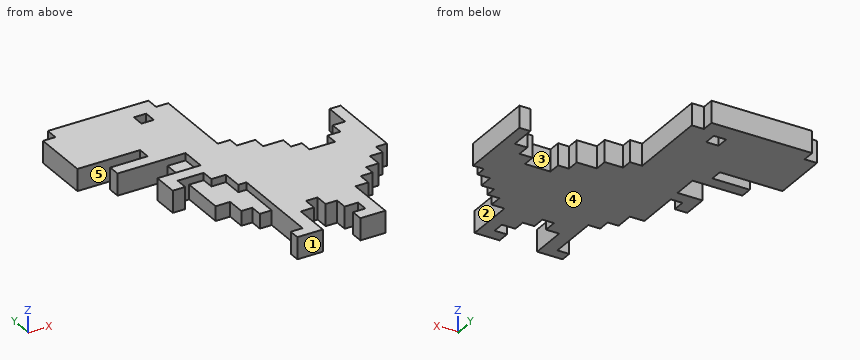
Autodesk Fusion 360 part; units mm, degrees
sketch "Dino" plane through (0, 0, 0) normal (0, 0, 1) x (1, 0, 0)
  line L0 (16.5, 0) -> (20, 0)
  line L1 (20, 0) -> (20, 5)
  line L2 (20, 5) -> (21.8166, 5)
  line L3 (21.8166, 5) -> (21.8166, 6.8132)
  line L4 (21.8166, 6.8132) -> (23.4038, 6.8132)
  line L5 (23.4038, 6.8132) -> (23.4038, 5)
  line L6 (23.4038, 5) -> (25, 5)
  line L7 (25, 5) -> (25, 3.315)
  line L8 (25, 3.315) -> (26.8534, 3.315)
  line L9 (26.8534, 3.315) -> (26.8534, 1.6631)
  line L10 (26.8534, 1.6631) -> (25.1529, 1.6631)
  line L11 (25.1529, 1.6631) -> (25.1529, 0)
  line L12 (25.1529, 0) -> (28.5781, 0)
  line L13 (28.5781, 0) -> (28.5781, 6.758)
  line L14 (28.5781, 6.758) -> (30.3565, 6.758)
  line L15 (30.3565, 6.758) -> (30.3565, 8.5127)
  line L16 (30.3565, 8.5127) -> (32, 8.5127)
  line L17 (32, 8.5127) -> (32, 10)
  line L18 (32, 10) -> (33.7351, 10)
  line L19 (33.7351, 10) -> (33.7351, 12)
  line L20 (33.7351, 12) -> (35.5, 12)
  line L21 (35.5, 12) -> (35.5, 13.5)
  line L22 (35.5, 13.5) -> (37, 13.5)
  line L23 (37, 13.5) -> (37, 24)
  line L24 (37, 24) -> (35.5, 24)
  line L25 (35.5, 24) -> (35.5, 20.5)
  line L26 (35.5, 20.5) -> (33.7869, 20.5)
  line L27 (33.7869, 20.5) -> (33.7869, 18.75)
  line L28 (33.7869, 18.75) -> (32, 18.75)
  line L29 (32, 18.75) -> (32, 17.0258)
  line L30 (32, 17.0258) -> (28.5, 17.0258)
  line L31 (28.5, 17.0258) -> (28.5, 18.75)
  line L32 (28.5, 18.75) -> (27, 18.75)
  line L33 (27, 18.75) -> (27, 20.5)
  line L34 (27, 20.5) -> (24.2282, 20.5)
  line L35 (24.2282, 20.5) -> (24.2282, 22.2618)
  line L36 (24.2282, 22.2618) -> (21.6914, 22.2618)
  line L37 (21.6914, 22.2618) -> (21.6914, 23.7839)
  line L38 (21.6914, 23.7839) -> (20, 23.7839)
  line L39 (20, 23.7839) -> (20, 35)
  line L40 (20, 35) -> (18.3225, 35)
  line L41 (18.3225, 35) -> (18.3225, 36.7116)
  line L42 (18.3225, 36.7116) -> (4.5, 36.7116)
  line L43 (4.5, 36.7116) -> (4.5, 35)
  line L44 (4.5, 35) -> (2.7971, 35)
  line L45 (2.7971, 35) -> (2.7971, 27.2137)
  line L46 (2.7971, 27.2137) -> (11.4112, 27.2137)
  line L47 (11.4112, 27.2137) -> (11.4112, 25.5)
  line L48 (11.4112, 25.5) -> (6.2675, 25.5)
  line L49 (6.2675, 25.5) -> (6.2675, 23.8448)
  line L50 (6.2675, 23.8448) -> (13.127, 23.8448)
  line L51 (13.127, 23.8448) -> (13.127, 20.4572)
  line L52 (13.127, 20.4572) -> (9.6973, 20.4572)
  line L53 (9.6973, 20.4572) -> (9.6973, 17)
  line L54 (9.6973, 17) -> (11.4121, 17)
  line L55 (11.4121, 17) -> (11.4121, 18.7286)
  line L56 (11.4121, 18.7286) -> (13, 18.7286)
  line L57 (13, 18.7286) -> (13, 12.7374)
  line L58 (13, 12.7374) -> (15, 12.7374)
  line L59 (15, 12.7374) -> (15, 10.206)
  line L60 (15, 10.206) -> (16.5, 10.206)
  line L61 (16.5, 10.206) -> (16.5, 8.5)
  line L62 (16.5, 8.5) -> (18.1296, 8.5)
  line L63 (18.1296, 8.5) -> (18.1296, 1.5)
  line L64 (18.1296, 1.5) -> (16.5, 1.5)
  line L65 (16.5, 1.5) -> (16.5, 0)
  line L66 (13.127, 23.8448) -> (15.6157, 23.8448)
  line L67 (15.6157, 23.8448) -> (15.6157, 20.4572)
  line L68 (15.6157, 20.4572) -> (13.127, 20.4572)
  line L69 (13, 18.7286) -> (15, 18.7286)
  line L70 (15, 18.7286) -> (15, 17)
  line L71 (15, 17) -> (17, 17)
  line L72 (17, 17) -> (17, 14.1994)
  line L73 (17, 14.1994) -> (18.1296, 14.1994)
  line L74 (18.1296, 14.1994) -> (18.1296, 8.5)
  line L75 (14.802, 34.2204) -> (14.802, 32.5)
  line L76 (14.802, 32.5) -> (16.5, 32.5)
  line L77 (16.5, 32.5) -> (16.5, 34.2204)
  line L78 (16.5, 34.2204) -> (14.802, 34.2204)
extrude "Extrude1" add sketch "Dino" along normal blind 3 contours L0 L1 L2 L3 L4 L5 L6 L7 L8 L9 L10 L11 L12 L13 L14 L15 L16 L17 L18 L19 L20 L21 L22 L23 L24 L25 L26 L27 L28 L29 L30 L31 L32 L33 L34 L35 L36 L37 L38 L39 L40 L41 L42 L43 L44 L45 L46 L47 L48 L49 L50 L52 L53 L54 L55 L56 L63 L64 L65 L66 L67 L68 L69 L70 L71 L72 L73 L74
extrude "Extrude2" add sketch "Dino" along normal blind 2 contours L57 L58 L59 L60 L61 L62 L69 L70 L71 L72 L73 L74 | L51 L66 L67 L68
For this review, take the finished solid that the model builds, in its own axes (mm). Face numbers are marked on the shaded views. A direction names the side the tool comes from. Round coordinates to 2 decimals unless told otherwise and drop trailing zeros. Loops run counter-clockwise (first coordinate to the right, second up) from the corner with the lowest first, then second, coordinate; pieces in that order, holes last. Notation, with made-up numbers: (-2.5, 55.5) - (55.5, 55.5) arc R31 cw to (55.5, 92.5) - close; hole circle Ø9 at (74, 51.5). An arc over 180 degrees is marked (long way). Put each result on its own line as item: value. Start each with the question number.
1. Consider section B-B on y = 33.5. State the section outline as (x, z) points, plus the area to 3 significant figures.
2. For the marked faces 1, 2, 3, 4 and 5, list the 3-axis set-ups (+Z, -Z, +X, -X, +Y, -Y) from which the entire face can be reached by the end or side of a thin tool; tool diameter is ignored.
3. Consider section A-A on x = 8. State the section outline as (y, z) points.
4. Insertion check: P1, Ø1.1, axis at x = 15.5, z = 2.5, coming from the -Y side; P2, Ø1, axis at y = 28, z = 2, coming from the +X side; P3, Ø1, axis at y = 6, z = 1, coming from the +X side. Each pin has a flat end and moves straight along its axis. Give the tip position at first contact, or say it passes through.
5. Consider section D-D on y = 23. State the section outline as (x, z) points.
6. Consider section C-C on y = 18. State the section outline as (x, z) points, plus the area to 3 significant figures.
7. For probe 1 along X at (y, z) = (21.5, 0.7); probe 2 along X at (y, z) = (34, 1); probe 3 along Y at (x, z) = (7.5, 1.8), list the stretches that pass through material, from the lowest coordinate up. Write a range as [from, to].
Result sheet:
1. outline: (2.8, 0) - (14.8, 0) - (14.8, 3) - (2.8, 3) - close; (16.5, 0) - (20, 0) - (20, 3) - (16.5, 3) - close
1. area: 46.5 mm^2
2. face 1: +Z, -Z, +X, -X, -Y
2. face 2: +Z, -Z, +X, -Y
2. face 3: +Z, -Z, +Y
2. face 4: -Z, +X, -X, +Y, -Y
2. face 5: +Z, -Z, -X
3. outline: (23.84, 0) - (25.5, 0) - (25.5, 3) - (23.84, 3) - close; (27.21, 0) - (36.71, 0) - (36.71, 3) - (27.21, 3) - close
4. P1: y = 10.21
4. P2: x = 20
4. P3: x = 28.58
5. outline: (13.13, 0) - (21.69, 0) - (21.69, 3) - (15.62, 3) - (15.62, 2) - (13.13, 2) - close; (35.5, 0) - (37, 0) - (37, 3) - (35.5, 3) - close
6. outline: (9.7, 0) - (11.41, 0) - (11.41, 3) - (9.7, 3) - close; (13, 0) - (28.5, 0) - (28.5, 3) - (15, 3) - (15, 2) - (13, 2) - close; (32, 0) - (37, 0) - (37, 3) - (32, 3) - close
6. area: 64.6 mm^2
7. probe 1: [13.13, 24.23], [35.5, 37]
7. probe 2: [2.8, 14.8], [16.5, 20]
7. probe 3: [23.84, 25.5], [27.21, 36.71]
